Autodesk Inventor part; units mm, degrees
ref_plane "YZ Plane" through (0, 0, 0) normal (1, 0, 0) x (0, 1, 0)
ref_plane "XZ Plane" through (0, 0, 0) normal (0, 1, 0) x (-1, 0, 0)
ref_plane "XY Plane" through (0, 0, 0) normal (0, 0, 1) x (1, 0, 0)
sketch "Sketch4" plane through (0, 0, 0) normal (0, 0, 1) x (1, 0, 0)
  line L0 (-3.1, 0) -> (5, 0)
  line L1 (0, 0) -> (-3.1, 0)
  line L2 (0, 4) -> (0, 2.66)
  line L3 (0.7, 1.96) -> (0.7, 1.96)
  line L4 (0.7, 1.96) -> (1.4, 2)
  arc A0 (0, 2.66) -> (0.7, 1.96) centre (0.7, 2.66) ccw
  line L5 (-3.1, 0) -> (-3.1, 2)
  line L6 (0, 4) -> (-1.5716, 4)
  arc A1 (-1.5716, 4) -> (-3.1, 2) centre (2.731, -0.8721) ccw
  line L7 (1.4, 2) -> (5, 2)
  line L8 (5, 2) -> (5, 0)
  point P0 (0, 1.96)
  dimension "d71" = 0.7
  dimension "d72" = 5
  dimension "d74" = 0.7
  dimension "d75" = 3.92
  dimension "d78" = 4
  dimension "d82" = 6.5
  dimension "d83" = 3.1
  dimension "d84" = 8
  dimension "d104" = 3.6
  dimension "d105" = 4
revolve "Revolution7" add sketch "Sketch4" angle 360 about axis through (-3.1, 0, 0) along (1, 0, 0)
sketch "Sketch5" plane through (-3.1, 0, 0) normal (-1, 0, 0) x (0, 0, 1)
  circle A0 centre (0, 0) radius 1.975 construction
  circle A1 centre (0, 0) radius 1.3825 construction
  line L0 (0, 0) -> (-1.1973, 0.6912)
  line L1 (0, 0) -> (-1.1973, -0.6912)
  line L2 (-1.8008, 0) -> (1.7887, 0)
  line L3 (-1.975, 0) -> (-1.1973, -0.6912)
  line L4 (-1.975, 0) -> (-1.1973, 0.6912)
  point P0 (0, 0)
  dimension "d88" = 3.95
  dimension "d89" = 2.765
  dimension "d90" = 30
  dimension "d91" = 30
extrude "Extrusion1" cut sketch "Sketch5" against normal blind 1.66
pattern_circular "Circular Pattern1" count 6 over 360 about axis through (-10, 0, 0) along (1, 0, 0) of "Extrusion1"
fillet "Fillet1" radius 0.395 12 edges at (-2.27, -1.7104, -0.9875) (-2.27, -0.6912, -1.1973) (-2.27, -1.3825, 0) (-2.27, -1.7104, 0.9875) (-2.27, -0.6912, 1.1973) (-2.27, 0, 1.975) (-2.27, 1.3825, 0) (-2.27, 1.7104, 0.9875) (-2.27, 0.6913, 1.1973) (-2.27, 0.6912, -1.1973) (-2.27, 0, -1.975) (-2.27, 1.7104, -0.9875)
thread "Thread7"
equation "\"a\" = 1.4"
equation "\"b\" = 3.6"
equation "\"dk\" = 8"
equation "\"k\" = 3.1"
equation "\"r\" = 0.7"
equation "\"rf\" = 6.5"
equation "\"x\" = 0.7"
equation "\"A_\" = 3.95"
equation "\"t\" = 1.66"
equation "\"p\" = 0.7"
equation "\"l_\" = 5"
equation "\"d\" = 4"
equation "\"ds_\" = 3.92"
equation "\"lg\" = 0"
properties part number "Flachkopfschraube mit Innenrund ISO 14583 - M4 x 5 - A2-70" material "Edelstahl"
Here's how the part is built. I have some questions about the finished solid (model axes, mm). A direction names the side the tool comes from. Round coordinates to 2 decimals unless told otherwise and drop trailing zeros. Order: outer loops, then holes, each group sorted by start corner. A loop starts at its lowest first (then second) coordinate and runs counter-clockwise, first axis right, second up. Notation, with made-up numbers: (-34.5, 10.25) -> (23.5, 10.25) arc R13 cw to (23.5, 23.25) -> close; hole circle Ø11 at (81.25, -24.5). An arc over 180 degrees is marked (long way). Return JSON: item names as keys, results as strings.
Q1. I need wall thicknesses on line 1 along Z through (x, y) = (-1.5, 0.25); line 2 along Y through (x, z) = (-2.5, -0.5); line 3 along Z through (x, y) = (-1.75, -0.5). Which ranges of each line are inside material? Lowest first, please. Write a range as from..to.
Filled sheet:
{"line 1": "z = -3.99..-1.69, 1.69..3.99", "line 2": "y = -2.94..-1.55, 1.55..2.94", "line 3": "z = -3.8..-1.41, 1.41..3.8"}
Q2. If we mould it in two halves opening along X, with no side actions, what happens to faces 1 (the flat face through (-1.44, 0, 0)), 2 (the cylindrical face through (-0.797, -0.867, 3.905)), 3 (the conical face through (0.977, 1.885, 0.593))? For each: released by +X, released by -X, zero draft, split by the parting line, or undercut.
Filled sheet:
{"face 1": "released by -X", "face 2": "zero draft", "face 3": "undercut"}
Q3. If we section it at A-A on x = 4: List the corners of the cut face in (y, z) for me.
Filled sheet:
{"outline": "circle Ø4 at (0, 0)"}
Q4. For pin 1 Ø1.5 at (x, y) = (2.5, -2) entering from -Z; pin 2 Ø4 at (x, y) = (-1.5, 1.5) entering from +Z, each with a flat end and sliding along its axis, tell me the tip position at first contact or that it passes through.
Filled sheet:
{"pin 1": "stops at z = -1.56", "pin 2": "stops at z = 4"}
Q5. Which directions (+Z, -Z, +X, -X, +Y, -Y) give clear straight access to the entire face, cutting with the end or side of a thin tool? Please do faces 4 (the flat face through (0, 3, -1)), 5 (the flat face through (5, 0, 0)).
Filled sheet:
{"face 4": "+X", "face 5": "+Z, -Z, +X, +Y, -Y"}
